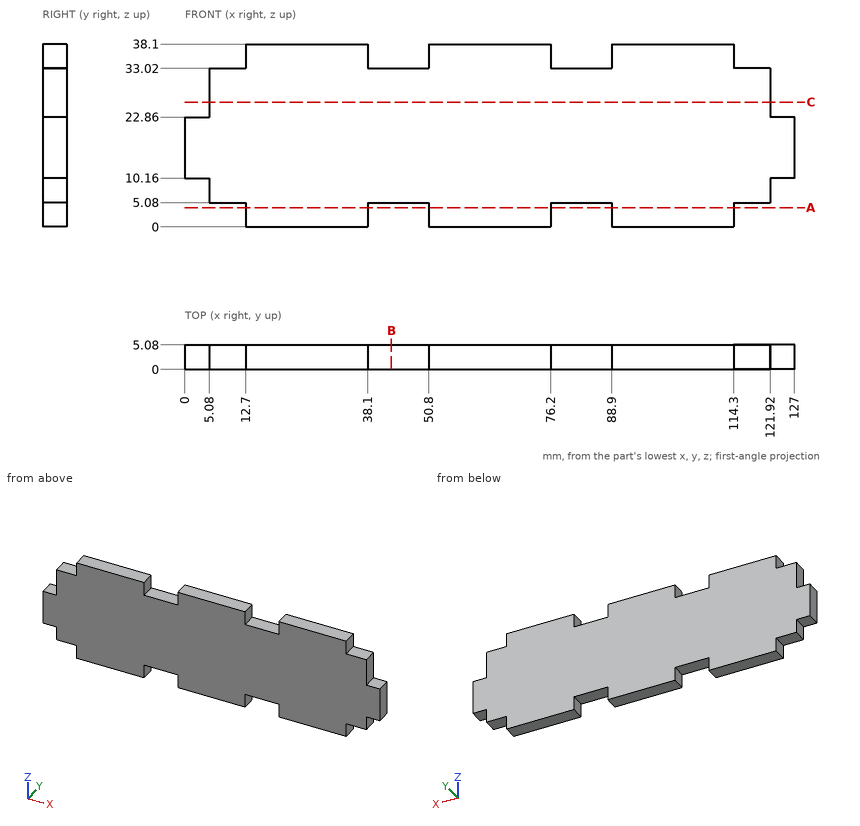
Can you work these out from the drawing? Everything is in mm from the part's minimum corner. Round coordinates to 2 decimals unless told otherwise and drop trailing zeros. Loops run counter-clockwise (first coordinate to the right, second up) from the corner with the lowest first, then second, coordinate; pieces in that order, holes last. Notation, with made-up numbers: (-4.5, -37.5) - (24.5, -37.5) arc R17 ccw to (24.5, -11.5) - close; hole circle Ø11 at (-39, 64). An arc over 180 degrees is marked (long way). Answer in a Markdown table with one row per item. Add a question column.
(1) If we section it at C-C (z = 26): Please give me the cut outline in (x, y), plus the area to 3 significant figures.
(2) If we section it at A-A (z = 4): Please give me the cut outline in (x, y).
(3) If we section it at B-B (x = 43): Please give me the cut outline in (y, z).
(4) I need wall thicknesses on line 1 along X through (y, z) = (0.45, 37); line 2 along Z through (x, y) = (10.5, 0.4); line 3 along X through (y, z) = (3.5, 8). Which ranges of each line are inside material? Lowest first, please.
(5) I'm going to push flat-ended pins straight in: pin 1 (1.5 mm diameter, centred on y = 2, z = 35, fed in from -X); pin 2 (1.5 mm diameter, centred on x = 118, y = 2, fed in from -Z); pin 3 (1.5 mm diameter, centred on x = 82, y = 2, fed in from +Z). Where does each tip first touch, or does it pass through?
Model answer:
| question | item | result |
|---|---|---|
| 1 | outline | (5.08, 0) - (121.92, 0) - (121.92, 5.08) - (5.08, 5.08) - close |
| 1 | area | 594 mm² |
| 2 | outline | (12.7, 0) - (38.1, 0) - (38.1, 5.08) - (12.7, 5.08) - close; (50.8, 0) - (76.2, 0) - (76.2, 5.08) - (50.8, 5.08) - close; (88.9, 0) - (114.3, 0) - (114.3, 5.08) - (88.9, 5.08) - close |
| 3 | outline | (0, 5.08) - (5.08, 5.08) - (5.08, 33.02) - (0, 33.02) - close |
| 4 | line 1 | x = 12.7 to 38.1, 50.8 to 76.2, 88.9 to 114.3 |
| 4 | line 2 | z = 5.08 to 33.02 |
| 4 | line 3 | x = 5.08 to 121.92 |
| 5 | pin 1 | stops at x = 12.7 |
| 5 | pin 2 | stops at z = 5.08 |
| 5 | pin 3 | stops at z = 33.02 |
